Autodesk Fusion 360 part; units mm, degrees
sketch "Sketch1" plane through (0, 0, 0) normal (0, 0, 1) x (1, 0, 0)
  line L0 (0, 0) -> (107, 0)
  line L1 (107, 0) -> (107, 67)
  line L2 (107, 67) -> (0, 67)
  line L3 (0, 67) -> (0, 0)
  line L4 (-3, 67) -> (-3, 70)
  line L5 (-3, 70) -> (0, 70)
  line L6 (110, 0) -> (110, -3)
  line L7 (110, -3) -> (107, -3)
  line L8 (-3, 70) -> (110, 70)
  line L9 (110, 70) -> (110, -3)
  line L10 (110, -3) -> (-3, -3)
  line L11 (-3, -3) -> (-3, 70)
  dimension "d1" = 67
  dimension "d2" = 107
  dimension "d3" = 3
  dimension "d4" = 3
  dimension "d5" = 3
extrude "Extrude1" add sketch "Sketch1" along normal blind 3
extrude "Extrude2" add sketch "Sketch1" along normal blind 3 contours L0 L1 L2 L3
fillet "Fillet1" radius 2.5 4 edges at (-3, 70, 1.5) (110, 70, 1.5) (110, -3, 1.5) (-3, -3, 1.5)
sketch "Sketch2" plane through (0, 0, 0) normal (0, 0, 1) x (1, 0, 0)
  line L0 (117.8476, 33.4729) -> (-7.2698, 33.4729)
  line L1 (53.5, 5) -> (53.5, 52.788)
  line L2 (0, 67) -> (0, 0)
  line L3 (2.75, 2.75) -> (2.75, 5.25)
  line L4 (2.75, 5.25) -> (0.25, 5.25)
  line L5 (0.25, 5.25) -> (0.25, 0.25)
  line L6 (0, 0) -> (107, 0)
  line L7 (0.25, 0.25) -> (5.25, 0.25)
  line L8 (5.25, 0.25) -> (5.25, 2.75)
  line L9 (5.25, 2.75) -> (2.75, 2.75)
  line L10 (5.25, 66.6957) -> (5.25, 64.1957)
  line L11 (5.25, 64.1957) -> (2.75, 64.1957)
  line L12 (2.75, 64.1957) -> (2.75, 61.6957)
  line L13 (2.75, 61.6957) -> (0.25, 61.6957)
  line L14 (0.25, 61.6957) -> (0.25, 66.6957)
  line L15 (0.25, 66.6957) -> (5.25, 66.6957)
  line L16 (101.75, 0.25) -> (101.75, 2.75)
  line L17 (106.75, 0.25) -> (101.75, 0.25)
  line L18 (106.75, 5.25) -> (106.75, 0.25)
  line L19 (104.25, 5.25) -> (106.75, 5.25)
  line L20 (104.25, 2.75) -> (104.25, 5.25)
  line L21 (101.75, 2.75) -> (104.25, 2.75)
  line L22 (101.75, 64.1957) -> (104.25, 64.1957)
  line L23 (101.75, 66.6957) -> (101.75, 64.1957)
  line L24 (106.75, 66.6957) -> (101.75, 66.6957)
  line L25 (106.75, 61.6957) -> (106.75, 66.6957)
  line L26 (104.25, 61.6957) -> (106.75, 61.6957)
  line L27 (104.25, 64.1957) -> (104.25, 61.6957)
  line L28 (0.25, 5.25) -> (10.25, 5.25)
  line L29 (10.25, 5.25) -> (10.25, 12.25)
  line L30 (10.25, 12.25) -> (0.25, 12.25)
  line L31 (0.25, 12.25) -> (0.25, 5.25)
  line L32 (0.25, 61.6957) -> (10.25, 61.6957)
  line L33 (10.25, 61.6957) -> (10.25, 54.6957)
  line L34 (10.25, 54.6957) -> (0.25, 54.6957)
  line L35 (0.25, 54.6957) -> (0.25, 61.6957)
  dimension "d14" = 53.5
  dimension "d16" = 5
  dimension "d17" = 0.25
  dimension "d19" = 5
  dimension "d55" = 10
  dimension "d56" = 7
  dimension "d57" = 10
  dimension "d58" = 7
extrude "Extrude3" add sketch "Sketch2" against normal blind 10 contours L3 L4 L5 L7 L8 L9 L28 | L10 L11 L12 L13 L14 L15 L32 | L16 L17 L18 L19 L20 L21 | L22 L23 L24 L25 L26 L27
fillet "Fillet2" radius 0.5 4 edges at (106.75, 0.25, -5) (106.75, 66.6957, -5) (0.25, 66.6957, -5) (0.25, 0.25, -5)
sketch "Sketch3" plane through (0, 0, 0) normal (0, 0, -1) x (1, 0, 0)
  line L0 (101.75, -0.25) -> (106.25, -0.25)
  arc A0 (106.75, -0.75) -> (106.25, -0.25) centre (106.25, -0.75) ccw
  line L1 (106.75, -0.75) -> (106.75, -5.25)
  line L2 (106.75, -5.25) -> (104.25, -5.25)
  line L3 (104.25, -5.25) -> (104.25, -2.75)
  line L4 (104.25, -2.75) -> (101.75, -2.75)
  line L5 (101.75, -2.75) -> (101.75, -0.25)
  line L6 (2.75, -2.75) -> (2.75, -5.25)
  line L7 (2.75, -5.25) -> (0.25, -5.25)
  line L8 (0.25, -5.25) -> (0.25, -0.75)
  arc A1 (0.75, -0.25) -> (0.25, -0.75) centre (0.75, -0.75) ccw
  line L9 (0.75, -0.25) -> (5.25, -0.25)
  line L10 (5.25, -0.25) -> (5.25, -2.75)
  line L11 (5.25, -2.75) -> (2.75, -2.75)
  line L12 (104.25, -61.6957) -> (106.75, -61.6957)
  line L13 (106.75, -61.6957) -> (106.75, -66.1957)
  arc A2 (106.25, -66.6957) -> (106.75, -66.1957) centre (106.25, -66.1957) ccw
  line L14 (106.25, -66.6957) -> (101.75, -66.6957)
  line L15 (101.75, -66.6957) -> (101.75, -64.1957)
  line L16 (101.75, -64.1957) -> (104.25, -64.1957)
  line L17 (104.25, -64.1957) -> (104.25, -61.6957)
  line L18 (0.25, -61.6957) -> (2.75, -61.6957)
  line L19 (2.75, -61.6957) -> (2.75, -64.1957)
  line L20 (2.75, -64.1957) -> (5.25, -64.1957)
  line L21 (5.25, -64.1957) -> (5.25, -66.6957)
  line L22 (5.25, -66.6957) -> (0.75, -66.6957)
  arc A3 (0.25, -66.1957) -> (0.75, -66.6957) centre (0.75, -66.1957) ccw
  line L23 (0.25, -66.1957) -> (0.25, -61.6957)
  arc A4 (-0.5, 3) -> (-3, 0.5) centre (-0.5, 0.5) ccw
  line L24 (-3, 0.5) -> (-3, -67.5)
  arc A5 (-3, -67.5) -> (-0.5, -70) centre (-0.5, -67.5) ccw
  line L25 (-0.5, -70) -> (107.5, -70)
  arc A6 (107.5, -70) -> (110, -67.5) centre (107.5, -67.5) ccw
  line L26 (110, -67.5) -> (110, 0.5)
  arc A7 (110, 0.5) -> (107.5, 3) centre (107.5, 0.5) ccw
  line L27 (107.5, 3) -> (-0.5, 3)
  line L28 (8, -19.25) -> (100.5, -19.25)
  line L29 (100.5, -19.25) -> (100.5, -47.75)
  line L30 (100.5, -47.75) -> (8, -47.75)
  line L31 (8, -47.75) -> (8, -19.25)
  line L32 (54.25, -19.25) -> (54.25, 3)
  line L33 (54.25, -47.75) -> (54.25, -70)
  line L34 (102.5, -47.75) -> (102.5, -50.75)
  line L35 (102.5, -50.75) -> (100.5, -50.75)
  line L36 (5, -19.5) -> (5, -16.25)
  line L37 (5, -16.25) -> (8, -16.25)
  line L38 (5, -16.25) -> (102.5, -16.25)
  line L39 (102.5, -16.25) -> (102.5, -50.75)
  line L40 (102.5, -50.75) -> (5, -50.75)
  line L41 (5, -50.75) -> (5, -16.25)
  dimension "d25" = 28.5
  dimension "d26" = 92.5
  dimension "d27" = 7.75
  dimension "d28" = 2
  dimension "d29" = 3
  dimension "d30" = 3
extrude "Extrude4" cut sketch "Sketch3" against normal blind 5 contours L28 L29 L30 L31
extrude "Extrude5" add sketch "Sketch3" along normal blind 10.5 contours L28 L29 L30 L32 L33 L34 L35 L38 L39 L40 | L28 L30 L31 L32 L33 L36 L37 L38 L40 L41
sketch "Sketch4" plane through (0, 0, -10.5) normal (0, 0, -1) x (1, 0, 0)
  line L0 (100.5, -47.75) -> (8, -47.75)
  line L1 (8, -47.75) -> (8, -19.25)
  line L2 (8, -19.25) -> (100.5, -19.25)
  line L3 (100.5, -19.25) -> (100.5, -47.75)
  line L4 (5, -50.75) -> (102.5, -50.75)
  line L5 (102.5, -50.75) -> (102.5, -16.25)
  line L6 (102.5, -16.25) -> (5, -16.25)
  line L7 (5, -16.25) -> (5, -50.75)
  circle A0 centre (11.835, -22.64) radius 0.575
  circle A1 centre (96.665, -22.64) radius 0.575
  circle A2 centre (96.665, -44.36) radius 0.575
  circle A3 centre (11.835, -44.36) radius 0.575
  line L8 (12.41, -22.64) -> (15.335, -22.64)
  line L9 (15.335, -22.64) -> (15.335, -26.14)
  line L10 (15.335, -26.14) -> (11.835, -26.14)
  line L11 (11.835, -26.14) -> (11.835, -23.215)
  line L12 (12.41, -44.36) -> (15.335, -44.36)
  line L13 (15.335, -44.36) -> (15.335, -40.86)
  line L14 (15.335, -40.86) -> (11.835, -40.86)
  line L15 (11.835, -40.86) -> (11.835, -43.785)
  line L16 (96.09, -44.36) -> (93.165, -44.36)
  line L17 (93.165, -44.36) -> (93.165, -40.86)
  line L18 (93.165, -40.86) -> (96.665, -40.86)
  line L19 (96.665, -40.86) -> (96.665, -43.785)
  line L20 (96.09, -22.64) -> (93.165, -22.64)
  line L21 (93.165, -22.64) -> (93.165, -26.14)
  line L22 (93.165, -26.14) -> (96.665, -26.14)
  line L23 (96.665, -26.14) -> (96.665, -23.215)
  line L24 (93.165, -26.14) -> (100.5, -26.14)
  line L25 (100.5, -26.14) -> (100.5, -19.25)
  line L26 (100.5, -19.25) -> (93.165, -19.25)
  line L27 (93.165, -19.25) -> (93.165, -26.14)
  line L28 (93.165, -40.86) -> (100.5, -40.86)
  line L29 (100.5, -40.86) -> (100.5, -47.75)
  line L30 (100.5, -47.75) -> (93.165, -47.75)
  line L31 (93.165, -47.75) -> (93.165, -40.86)
  line L32 (15.335, -40.86) -> (8, -40.86)
  line L33 (8, -40.86) -> (8, -47.75)
  line L34 (8, -47.75) -> (15.335, -47.75)
  line L35 (15.335, -47.75) -> (15.335, -40.86)
  line L36 (15.335, -26.14) -> (8, -26.14)
  line L37 (8, -26.14) -> (8, -19.25)
  line L38 (8, -19.25) -> (15.335, -19.25)
  line L39 (15.335, -19.25) -> (15.335, -26.14)
  dimension "d36" = 84.83
  dimension "d39" = 1.15
  dimension "d40" = 1.15
  dimension "d41" = 1.15
  dimension "d42" = 1.15
  dimension "d43" = 3.5
  dimension "d44" = 3.5
  dimension "d45" = 3.5
  dimension "d46" = 3.5
  dimension "d47" = 3.5
  dimension "d48" = 3.5
  dimension "d49" = 3.5
  dimension "d50" = 3.5
extrude "Extrude6" add sketch "Sketch4" against normal blind 3 contours L0 L3 A2 L16 L19 L28 L29 L30 L31 | L0 L1 A3 L12 L15 L32 L33 L34 L35 | A2 L16 L17 L18 L19 L28 L31 | L2 L3 A1 L20 L23 L24 L25 L26 L27 | A3 L12 L13 L14 L15 L32 L35 | A1 L20 L21 L22 L23 L24 L27 | L1 L2 A0 L8 L11 L36 L37 L38 L39 | A0 L8 L9 L10 L11 L36 L39
fillet "Fillet3" radius 0.5 4 edges at (54.25, 19.25, 3) (54.25, 47.75, 3) (8, 33.5, 3) (100.5, 33.5, 3)
extrude "Extrude7" add sketch "Sketch2" against normal blind 7 contours L4 L28 L29 L30 L31 | L13 L32 L33 L34 L35
sketch "Sketch5" plane through (0.25, 0, 0) normal (-1, 0, 0) x (0, -1, 0)
  line L0 (-0.75, -10) -> (-0.75, 0)
  line L1 (-0.75, 0) -> (-12.25, 0)
  line L2 (-12.25, 0) -> (-12.25, -7)
  line L3 (-12.25, -7) -> (-5.25, -7)
  line L4 (-5.25, -7) -> (-5.25, -10)
  line L5 (-5.25, -10) -> (-0.75, -10)
  circle A0 centre (-8.625, -3.5) radius 5.0389
  circle A1 centre (-8.625, -3.5) radius 1.75
  circle A2 centre (-58.35, -3.5) radius 5.0569
  circle A3 centre (-58.35, -3.5) radius 1.75
  dimension "d61" = 3.5
  dimension "d62" = 3.5
extrude "Extrude8" cut sketch "Sketch5" against normal blind 7 contours A1 | A3
chamfer "Chamfer1" distance 0.8 angle 45 8 edges at (110, 33.5, 3) (109.2678, 69.2678, 3) (53.5, 70, 3) (-2.2678, 69.2678, 3) (-3, 33.5, 3) (-2.2678, -2.2678, 3) (53.5, -3, 3) (109.2678, -2.2678, 3)
equation "d14 = ( 107 / 2 ) * 1 mm"
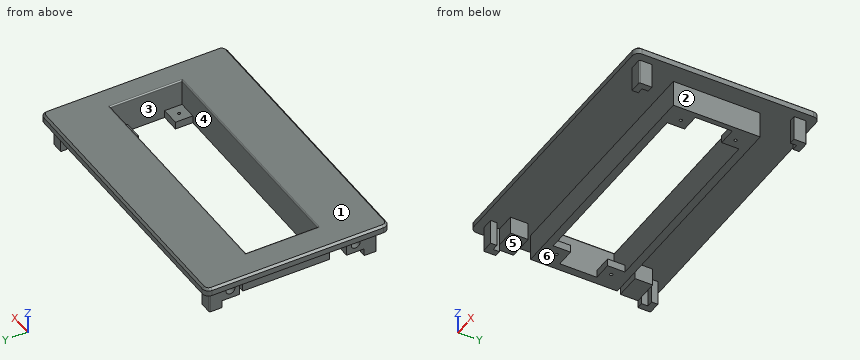
Geometry check sheet. Reference: the model listing, model coordinates, mm. Face numbers are marked on the shaded views. A direction names the side the tool comes from. Give positions to 0.01 mm unless a question says otherwise; leave off trailing zeros. Order: outer loops, then holes, each group sorted by start corner. A loop starts at its lowest first (then second) coordinate and runs counter-clockwise, first axis right, second up.
1. Draft check along X on the marked faces 1, 2 and 3. Enter one of: pulls with the +X half, pulls with the -X half, needs draft (parallel to the pull), parting line crosses it, or undercut.
Completed:
face 1: needs draft
face 2: pulls with the +X half
face 3: undercut
2. Scan lines: line 1 (X direction, y = 22.64, z = -9.1) (3 decimals); line 2 (Y direction, x = 64.5, z = -0.75); line 3 (Y direction, x = 105, z = -5.25). Record each from-to range of solid material in increasing order.
Completed:
line 1: x = 5 to 11.26, 12.41 to 15.335, 93.165 to 96.09, 97.24 to 102.5
line 2: y = 16.25 to 19.25, 47.75 to 50.75
line 3: y = 0.25 to 5.25, 61.7 to 66.7
3. Access from +Z, -Z, +X, -X, +Y, -Y to the whole of each face (thin tool, end or side, straight path). Record for the marked faces 4, 5 and 6.
Completed:
face 4: +Z
face 5: -Z, +X, -X
face 6: -Z, +X, -X, +Y, -Y
4. Sectioned sample at B-B (y = 38). Record the boundary of the cut face in (x, z), then the cut area to 3 significant figures.
Completed:
outline: (-3, 0) - (5, 0) - (5, -10.5) - (8, -10.5) - (8, 2.5) arc R0.5 ccw to (7.5, 3) - (-2.2, 3) - (-3, 2.2) - close; (100.5, -10.5) - (102.5, -10.5) - (102.5, 0) - (110, 0) - (110, 2.2) - (109.2, 3) - (101, 3) arc R0.5 ccw to (100.5, 2.5) - close
area: 113 mm2
5. Depth check by flat-ended pin: pin 1 (6.5 mm diameter, centred on y = 29, z = -4.5, fed in from -X); pin 2 (5 mm diameter, centred on x = 66, z = -7, fed in from -Y); pin 3 (6 mm diameter, centred on x = 84.5, z = -0.5, fed in from -Y); pin 4 (3 mm diameter, centred on x = 102.5, z = -6.5, fed in from -Y). Enter the tip coordinate at first touch or a pass-through.
Completed:
pin 1: stops at x = 5
pin 2: stops at y = 16.25
pin 3: stops at y = -3
pin 4: stops at y = 0.25
6. Sectioned sample at D-D (z = -3.5). State how many separate pieces and enclosed holes the cut face has, then the cut area to 3 significant figures.
Completed:
separate pieces: 5
enclosed holes: 1
area: 893 mm2
7. Sectioned sample at C-C (y = 49.5). Record the boundary of the cut face in (x, z), then the cut area to 3 significant figures.
Completed:
outline: (-3, 0) - (5, 0) - (5, -10.5) - (102.5, -10.5) - (102.5, 0) - (110, 0) - (110, 2.2) - (109.2, 3) - (-2.2, 3) - (-3, 2.2) - close
area: 1,360 mm2
8. Sectioned sample at A-A (x = 60). Record the boundary of the cut face in (y, z), then the cut area to 3 significant figures.
Completed:
outline: (-3, 0) - (16.25, 0) - (16.25, -10.5) - (19.25, -10.5) - (19.25, 2.5) arc R0.5 ccw to (18.75, 3) - (-2.2, 3) - (-3, 2.2) - close; (47.75, -10.5) - (50.75, -10.5) - (50.75, 0) - (70, 0) - (70, 2.2) - (69.2, 3) - (48.25, 3) arc R0.5 ccw to (47.75, 2.5) - close
area: 196 mm2
